The drawing under review shows one solid part. Ordinate dimensions are in mm from its lowest x, y, z. A direction names the side the tool comes from. Give positions to 0.01 mm unless a question says otherwise; leave off trailing zeros. Order: outer loops, then holes, each group sorted by start corner. A loop starts at its lowest first (then second) coordinate and runs counter-clockwise, first axis right, second up. Notation, with made-up numbers: (82, 79.25) -> (115, 79.25) arc R23 cw to (115, 108.25) -> close; hole circle Ø5 at (-36, 20.25). An arc over 180 degrees is marked (long way). One line per item, written item: value.
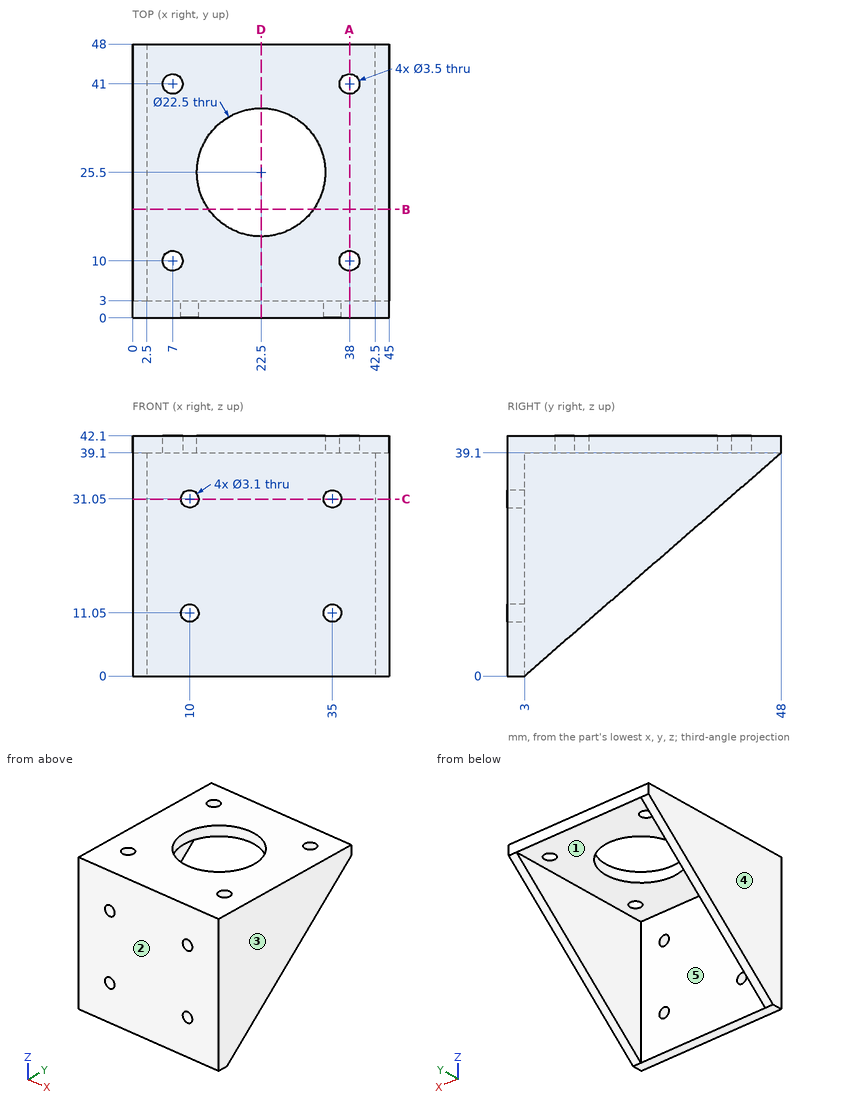
Item 1: To check wall thickness, follow line 1 along Y through (x, z) = (7, 41.35); line 2 along X through (y, z) = (2, 11); line 3 along X through (y, z) = (23, 30). State the ranges of each line that lie inside material, in increasing order. Write a range as from..to.
Returned:
line 1: 0..8.25, 11.75..39.25, 42.75..48
line 2: 0..8.45, 11.55..33.45, 36.55..45
line 3: 0..2.5, 42.5..45
Item 2: Machinability: for the marked faces 4 and 5, which of the approach directions +Z, -Z, +X, -X, +Y, -Y give a long, thin tool a straight path to every point of the face, cutting with its end or side? Answer none if there is none.
Returned:
face 4: +Z, -Z, -X, +Y, -Y
face 5: -Z, +Y
Item 3: Add section A-A on x = 38. Give the boundary of the cut face in (y, z), plus the area to 3 significant figures.
Returned:
outline: (0, 0) -> (3, 0) -> (3, 39.1) -> (8.25, 39.1) -> (8.25, 42.1) -> (0, 42.1) -> close; (11.75, 39.1) -> (39.25, 39.1) -> (39.25, 42.1) -> (11.75, 42.1) -> close; (42.75, 39.1) -> (48, 39.1) -> (48, 42.1) -> (42.75, 42.1) -> close
area: 240 mm²
Item 4: Draft analysis for pull direction X (two halves, no side actions). For the marked faces 1, 2 and 3, state which applies: pulls with the +X half, pulls with the -X half, needs draft (parallel to the pull), parting line crosses it, or undercut.
Returned:
face 1: undercut
face 2: needs draft
face 3: pulls with the +X half
Item 5: Add section C-C on z = 31. Give the boundary of the cut face in (x, y).
Returned:
outline: (0, 0) -> (8.45, 0) -> (8.45, 3) -> (2.5, 3) -> (2.5, 38.68) -> (0, 38.68) -> close; (11.55, 0) -> (33.45, 0) -> (33.45, 3) -> (11.55, 3) -> close; (36.55, 0) -> (45, 0) -> (45, 38.68) -> (42.5, 38.68) -> (42.5, 3) -> (36.55, 3) -> close
Item 6: Add section D-D on x = 22.5. Give the boundary of the cut face in (y, z).
Returned:
outline: (0, 0) -> (3, 0) -> (3, 39.1) -> (14.25, 39.1) -> (14.25, 42.1) -> (0, 42.1) -> close; (36.75, 39.1) -> (48, 39.1) -> (48, 42.1) -> (36.75, 42.1) -> close
Item 7: Clearance check with flat-ended pins moving along their axes: P1, Ø4.5, axis at x = 38, y = 41, coming from the -Z side; P2, Ø8, axis at x = 18.5, z = 7, coming from the +Y side. State where each tip first meets the part, or that it passes through.
Returned:
P1: z = 39.1
P2: y = 3
Item 8: Add section B-B on y = 19. Give the boundary of the cut face in (x, z).
Returned:
outline: (0, 13.9) -> (2.5, 13.9) -> (2.5, 39.1) -> (13.32, 39.1) -> (13.32, 42.1) -> (0, 42.1) -> close; (31.68, 39.1) -> (42.5, 39.1) -> (42.5, 13.9) -> (45, 13.9) -> (45, 42.1) -> (31.68, 42.1) -> close
